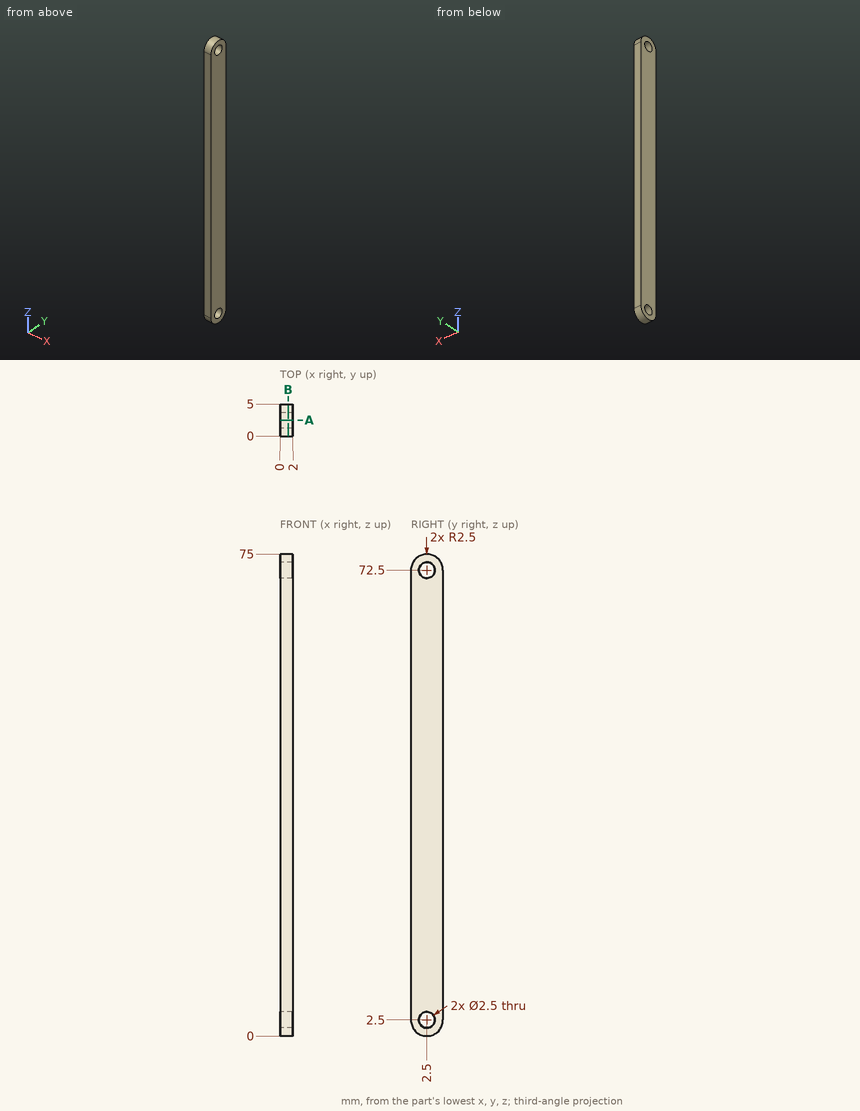
Input: dimensioned drawing with shaded views. Units: mm. Origin: part minimum x, y, z. Give positions to 0.01 mm unless a question says otherwise; leave off trailing zeros. Order: outer loops, then holes, each group sorted by start corner. A loop starts at its lowest first (then second) coordinate and runs counter-clockwise, first axis right, second up. Notation, with made-up numbers: (17, 12.5) -> (64, 12.5) arc R31 cw to (64, 38.5) -> close; hole circle Ø6 at (2, -5.5). An arc over 180 degrees is marked (long way). Write item = value, one per line.
Item 1: Section query B-B (x = 1.25). Output: boundary loops of the cut face in (y, z).
Check result:
outline = (0, 2.5) arc R2.5 ccw to (5, 2.5) -> (5, 72.5) arc R2.5 ccw to (0, 72.5) -> close; hole circle Ø2.5 at (2.5, 2.5); hole circle Ø2.5 at (2.5, 72.5)
Item 2: Section query A-A (y = 2.5). Output: boundary loops of the cut face in (x, z).
Check result:
outline = (0, 0) -> (2, 0) -> (2, 1.25) -> (0, 1.25) -> close; (0, 3.75) -> (2, 3.75) -> (2, 71.25) -> (0, 71.25) -> close; (0, 73.75) -> (2, 73.75) -> (2, 75) -> (0, 75) -> close
Item 3: Ray query, probe 1 along Z at (x, y) = (1.1, 2.5); probe 2 along Z at (x, y) = (1.8, 3.1); probe 3 along Y at (x, z) = (1.3, 72.5). Return the intervals inside material, ascending.
Check result:
probe_1 = 0 to 1.25, 3.75 to 71.25, 73.75 to 75
probe_2 = 0.07 to 1.4, 3.6 to 71.4, 73.6 to 74.93
probe_3 = 0 to 1.25, 3.75 to 5
Item 4: Contact query for a flat-ended pin moving along its axis: pin 1 (1.5 mm diameter, centred on y = 2.5, z = 2.5, fed in from -X). Output: stop coordinate, or through.
Check result:
pin_1 = through
